The model under review builds one solid part; all positions refer to its coordinate system, in mm. Face numbers are marked on the shaded views. A direction names the side the tool comes from. Give positions to 0.01 mm unless a question says otherwise; leave off trailing zeros. Loops run counter-clockwise (first coordinate to the right, second up) from the corner with the lowest first, then second, coordinate; pieces in that order, holes last. Notation, with made-up numbers: M 70.25,76.5 L 118.25,76.5 A15 ccw 118.25,103.5 Z; hole C 75,4.5 d4. An arc over 180 degrees is marked long. Put each result on its own line as item: value. Start each with the question number.
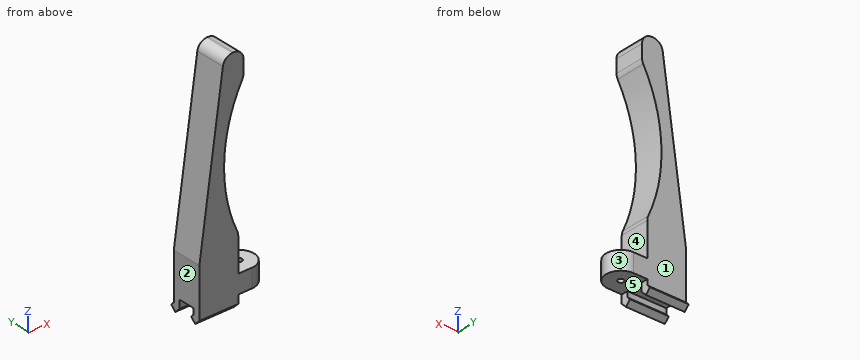
from build123d import *

# Parameters (mm, degrees)
SKETCH2_W           = 10
SKETCH2_H           = 14.768412439
BOSS_EXTRUDE1_DEPTH = 5
BOSS_EXTRUDE4_DEPTH = 10
SKETCH9_W           = 10
SKETCH9_H           = 3.18
SKETCH9_H_2         = 3.888412439
CUT_EXTRUDE3_DEPTH  = 5
BOSS_EXTRUDE5_DEPTH = 7.7
SKETCH12_R          = 0.75
BOSS_EXTRUDE7_DEPTH = 4.75
FILLET1_R           = 2.5


with BuildPart() as part:
    # Sketch2 → Boss-Extrude1 (new body)
    with BuildSketch(Plane.XY):
        with Locations((0, 1.566049366)):
            Rectangle(SKETCH2_W, SKETCH2_H)
    extrude(amount=BOSS_EXTRUDE1_DEPTH)

    # Sketch8 → Boss-Extrude4 (add)
    with BuildSketch(Plane.ZY.offset(5)):
        Polygon((-0.15, 5.770255585), (0, 5.770255585), (0, 4.070255585), (-0.15, 4.070255585), (-2.137867966, 4.070255585), (-3.402081528, 5.334469147), (-2.2, 6.536550675), (-1.43370491, 5.770255585), align=None)
        Polygon((-0.15, -1.929744415), (0, -1.929744415), (0, -0.229744415), (-0.15, -0.229744415), (-1.43370491, -0.229744415), (-2.2, 0.536550675), (-3.402081528, -0.665530853), (-2.137867966, -1.929744415), align=None)
    extrude(amount=-BOSS_EXTRUDE4_DEPTH)

    # Sketch9 → Cut-Extrude3 (cut)
    with BuildSketch(Plane(origin=(0, 0, 0), x_dir=(-1, 0, 0), z_dir=(0, 0, -1))):
        with Locations((0, 7.360255585)):
            Rectangle(SKETCH9_W, SKETCH9_H)
        with Locations((0, -3.873950635)):
            Rectangle(SKETCH9_W, SKETCH9_H_2)
    extrude(amount=-CUT_EXTRUDE3_DEPTH, mode=Mode.SUBTRACT)

    # Sketch10 → Boss-Extrude5 (add)
    with BuildSketch(Plane(origin=(0, 5.770255585, 0), x_dir=(1, 0, 0), z_dir=(0, 1, 0))):
        with BuildLine():
            Line((-5, -5), (-5, -10.5))
            Line((-5, -10.5), (1.352445729, -55.7))
            Line((1.352445729, -55.7), (6.352445729, -55.7))
            Line((6.352445729, -55.7), (6.352445729, -49.2))
            ThreePointArc((6.352445729, -49.2), (1.383429579, -31.764936646), (5, -14))
            Line((5, -14), (5, -5))
            Line((5, -5), (-5, -5))
        make_face()
    extrude(amount=-BOSS_EXTRUDE5_DEPTH)

    # Sketch12 → Boss-Extrude7 (add)
    with BuildSketch(Plane.XY):
        with BuildLine():
            Line((5, 5.770255585), (8.5, 5.770255585))
            ThreePointArc((8.5, 5.770255585), (12.35, 1.920255585), (8.5, -1.929744415))
            Line((8.5, -1.929744415), (5, -1.929744415))
            Line((5, -1.929744415), (5, 5.770255585))
        make_face()
        with Locations((8.5, 1.920255585)):
            Circle(SKETCH12_R, mode=Mode.SUBTRACT)
    extrude(amount=BOSS_EXTRUDE7_DEPTH)

    # Fillet1
    fillet1_edges = [part.edges().sort_by_distance(p)[0] for p in [
        (6.352445729, 1.920255585, 49.2),
        (5, 1.920255585, 14),
        (1.352445729, 1.920255585, 55.7),
        (6.352445729, 1.920255585, 55.7),
    ]]
    fillet(fillet1_edges, radius=FILLET1_R)


solid = part.part
(1) We need section A-A, the plane y = 3.5. Write out the cut boundary in (x, z).
(2) Insertion check: pin 1 (4 mm diameter, centred on x = 6, y = 5.5, fed in from +Z); pin 2 (5 mm diameter, centred on x = -2, z = 21.5, fed in from +Y); pin 3 (2.5 mm diameter, centred on y = 5.5, z = -2.5, fed in from +X). Each pin has a flat end and moves straight along its axis. Give the tip position at first contact, or say it passes through.
(3) To check wall thickness, follow L1, parallel to Y at x = 8.5, z = 2.2; L2, parallel to Y at x = -1.5, z = 33; L3, parallel to Z at x = 7, y = -1. State the ranges of each line that lie inside material, in increasing order. Write a range as [from, to].
(4) For the marked faces 1 and 2, list the 3-axis set-ups (+Z, -Z, +X, -X, +Y, -Y) from which the entire face can be reached by the end or side of a thin tool; tool diameter is ignored.
(5) Draft analysis for pull direction Y (two halves, no side actions). For the marked faces 3, 4 and 5, state which applies: +Y half, -Y half, draft (parallel to the pull), parting line (faces both ways), or undercut.
(6) We need section B-B, the plane x = -3.25. Write out the cut boundary in (y, z).
(7) We need section C-C, the plane z = 11.5. Write out the cut boundary in (x, y), plus the area to 3 significant figures.
Check sheet entries:
1. outline: M -5,0 L 12.01,0 L 12.01,4.75 L 5,4.75 L 5,13.45 A2.5 ccw 4.78,14.48 A38.25 cw 6.05,48.65 A2.5 ccw 6.35,49.85 L 6.35,53.2 A2.5 ccw 3.85,55.7 L 3.53,55.7 A2.5 ccw 1.05,53.55 L -5,10.5 Z
2. pin 1: stops at z = 55.7
2. pin 2: stops at y = 5.77
2. pin 3: stops at x = 5
3. L1: y = [-1.93, 1.17], [2.67, 5.77]
3. L2: y = [-1.93, 5.77]
3. L3: z = [0, 4.75]
4. face 1: +Z, +X, -X, +Y
4. face 2: +Z, -Z, -X, +Y, -Y
5. face 3: parting line
5. face 4: draft
5. face 5: undercut
6. outline: M -1.93,-2.14 L -0.67,-3.4 L 0.54,-2.2 L -0.23,-1.43 L -0.23,0 L 4.07,0 L 4.07,-2.14 L 5.33,-3.4 L 6.54,-2.2 L 5.77,-1.43 L 5.77,22.95 L -1.93,22.95 Z
7. outline: M -4.86,-1.93 L 5,-1.93 L 5,5.77 L -4.86,5.77 Z
7. area: 75.9 mm²
